```python
from build123d import *

# Parameters (mm, degrees)
CROQUIS1_W              = 28
CROQUIS1_H              = 32
CROQUIS1_R              = 3.96875
SALIENTE_EXTRUIR1_DEPTH = 6.35
REDONDEO1_R             = 10


with BuildPart() as part:
    # Croquis1 → Saliente-Extruir1 (new body)
    with BuildSketch(Plane.XY):
        with Locations((14, -16)):
            Rectangle(CROQUIS1_W, CROQUIS1_H)
        with Locations((14, -24)):
            Circle(CROQUIS1_R, mode=Mode.SUBTRACT)
    extrude(amount=SALIENTE_EXTRUIR1_DEPTH)

    # Redondeo1
    redondeo1_edges = [part.edges().sort_by_distance(p)[0] for p in [
        (28, -32, 3.175),
        (0, -32, 3.175),
    ]]
    fillet(redondeo1_edges, radius=REDONDEO1_R)


solid = part.part
```
CAD build for the part. Positions are in the model's coordinates, mm. Coordinates: 2 decimals unless noted, no trailing zeros. Order: outer loops, then holes, each group sorted by start corner. A loop starts at its lowest first (then second) coordinate and runs counter-clockwise, first axis right, second up. Notation, with made-up numbers: (86, 58.25) - (138, 58.25) arc R27 cw to (138, 94.25) - close; hole circle Ø2 at (-37.75, -9). An arc over 180 degrees is marked (long way). Use a Markdown table: item, result. Add a question column.
(1) Pull direction Y, two halves, no side cores. Call faces 1 (the face through (13.14, -27.874, 3.131)), 2 (the face through (14, 0, 3)), 3 (the face through (14, -16, 6.35)): +Y half, -Y half, draft (parallel to the pull), parting line (faces both ways), or undercut.
(2) Saw through at A-A (x = 14). Give the cut face in (y, z).
(3) Drill centre lines: line 1 along Y through (x, z) = (14, 5); line 2 along X through (y, z) = (-22, 6.25); line 3 along Y through (x, z) = (12.75, 5). Where is each one in solid material? Low to high. Write a range as [from, to].
(4) Saw through at C-C (z = 3.25). Give the cut face in (x, y).
(5) Flat gauge pin, fed straight in: pin 1 (5 mm diameter, centred on x = 14, y = -24, fed in from -Z). Where does the tip first touch, or does it go through?
(6) Saw through at D-D (x = 25). Give the cut face in (y, z).
(7) Saw through at B-B (y = -24.5). Give the cut face in (x, z), then the cut area to 3 significant figures.
Solved:
| question | item | result |
|---|---|---|
| 1 | face 1 | undercut |
| 1 | face 2 | +Y half |
| 1 | face 3 | draft |
| 2 | outline | (-32, 0) - (-27.97, 0) - (-27.97, 6.35) - (-32, 6.35) - close; (-20.03, 0) - (0, 0) - (0, 6.35) - (-20.03, 6.35) - close |
| 3 | line 1 | y = [-32, -27.97], [-20.03, 0] |
| 3 | line 2 | x = [0, 10.57], [17.43, 28] |
| 3 | line 3 | y = [-32, -27.77], [-20.23, 0] |
| 4 | outline | (0, -22) arc R10 ccw to (10, -32) - (18, -32) arc R10 ccw to (28, -22) - (28, 0) - (0, 0) - close; hole circle Ø7.94 at (14, -24) |
| 5 | pin 1 | passes through |
| 6 | outline | (-29.14, 0) - (0, 0) - (0, 6.35) - (-29.14, 6.35) - close |
| 7 | outline | (0.32, 0) - (10.06, 0) - (10.06, 6.35) - (0.32, 6.35) - close; (17.94, 0) - (27.68, 0) - (27.68, 6.35) - (17.94, 6.35) - close |
| 7 | area | 124 mm² |
